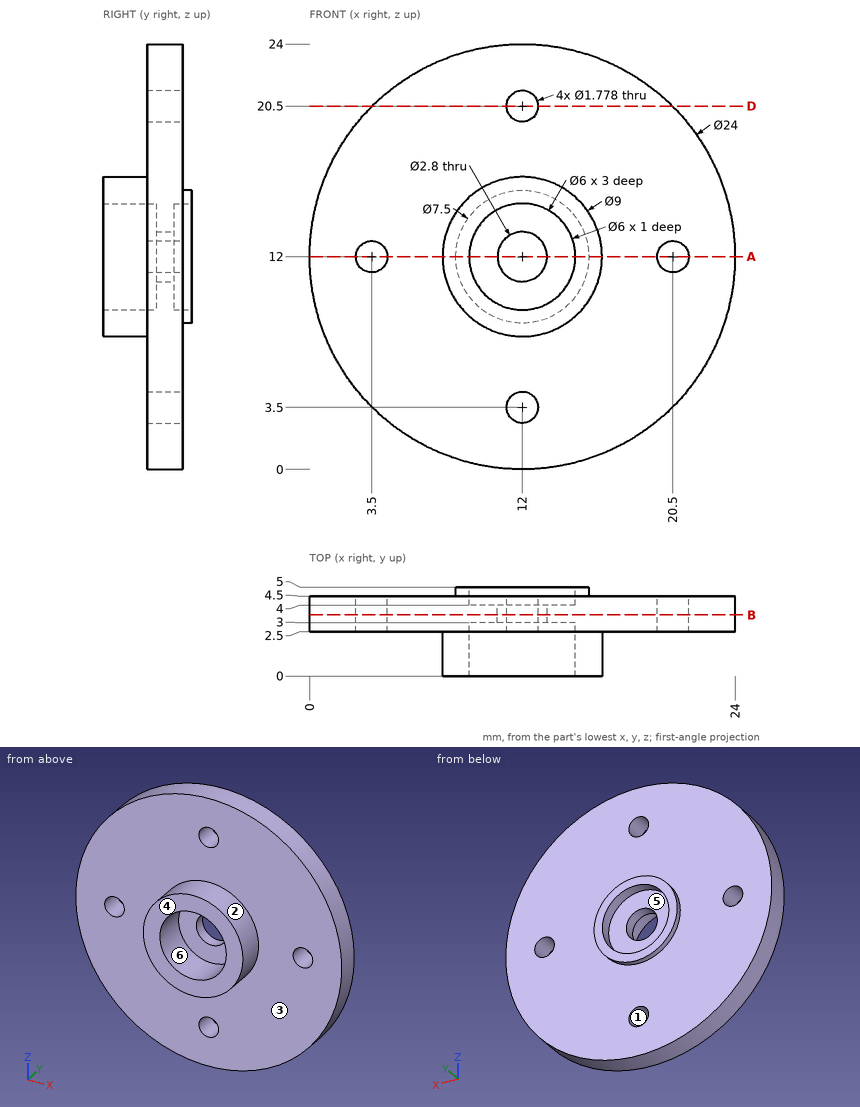
Verification items for this drawing (mm, ordinates from the low corner). A direction names the side the tool comes from. Coordinates: 2 decimals unless noted, no trailing zeros. Write each loop counter-clockwise with the first axis right and the second up, starting at its lowest first coordinate (ties: lowest second). Pieces come first, ordered by that corner, then holes. Notation, with made-up numbers: M 26,-38 L 47,-38 A19 ccw 47,-12 Z; hole C -16.5,72.25 d4. An arc over 180 degrees is marked long. Use one line per item in the form item = value. Start each with the question number.
1) Thickness scan on probe 1 along Z at (x, y) = (12, 3.45); probe 2 along Z at (x, y) = (12, 2.25); probe 3 along X at (y, z) = (2.65, 11.75). Record the ranges inside material, lowest first. Write a range as from..to.
2) Set-up check for the marked faces 4, 5 and 6: record each of +Z, -Z, +X, -X, +Y, -Y from which the full face is reachable in a straight line by a thin tool's end or side.
3) Section check A-A on z = 12. State how many separate pieces and enclosed holes the cut face has, and give its area (3 significant figures).
4) Go/stop test with flat-tipped pins: pin 1 Ø1.5 at (x, y) = (8, 2) entering from -Z; pin 2 Ø2.5 at (x, z) = (20.5, 12) entering from +Y; pin 3 Ø6.5 at (x, z) = (11.5, 12) entering from -Y; pin 4 Ø3.5 at (x, z) = (12, 12) entering from +Y. Record where each tip stops, or that it passes through.
5) Section check D-D on z = 20.5. Enter the section's corners in (x, y).
6) Section check B-B on y = 3.45. Enter the section's corners in (x, z), and give its area (3 significant figures).
7) Release check for a two-part mould opening along X. For the marked faces 1, 2 and 3 record: pulls with the +X half, pulls with the -X half, needs draft (parallel to the pull), parting line crosses it, or undercut.
Responses:
q1.probe_1 = 0..2.61, 4.39..10.6, 13.4..19.61, 21.39..24
q1.probe_2 = 7.5..9, 15..16.5
q1.probe_3 = 0..2.65, 4.35..9.01, 14.99..19.65, 21.35..24
q2.face_4 = +Z, -Z, +X, -X, -Y
q2.face_5 = +Y
q2.face_6 = -Y
q3.separate_pieces = 4
q3.enclosed_holes = 0
q3.area = 40.3 mm2
q4.pin_1 = 0.5
q4.pin_2 = 4.5
q4.pin_3 = 0
q4.pin_4 = 4
q5.outline = M 3.53,2.5 L 11.11,2.5 L 11.11,4.5 L 3.53,4.5 Z; M 12.89,2.5 L 20.47,2.5 L 20.47,4.5 L 12.89,4.5 Z
q6.outline = C 12,12 d24; hole C 3.5,12 d1.78; hole C 12,12 d2.8; hole C 12,3.5 d1.78; hole C 12,20.5 d1.78; hole C 20.5,12 d1.78
q6.area = 436 mm2
q7.face_1 = undercut
q7.face_2 = parting line crosses it
q7.face_3 = needs draft
